from build123d import *

# Parameters (mm, degrees)
F0_R     = 29
F0_R_2   = 20.25
F1_DEPTH = 40
F2_SIZE  = 5
F3_SIZE  = 2
F4_SIZE  = 2
F5_SIZE  = 5


with BuildPart() as f1:
    # F0 (on Top) → F1 (new body, symmetric)
    with BuildSketch(Plane.XY):
        Circle(F0_R)
        Circle(F0_R_2, mode=Mode.SUBTRACT)
    extrude(amount=F1_DEPTH, both=True)

    # F2
    f2_edges = [f1.edges().sort_by_distance(p)[0] for p in [
        (-20.25, 0, 40),
    ]]
    chamfer(f2_edges, length=F2_SIZE)

    # F3
    f3_edges = [f1.edges().sort_by_distance(p)[0] for p in [
        (-29, 0, -40),
    ]]
    chamfer(f3_edges, length=F3_SIZE)

    # F4
    f4_edges = [f1.edges().sort_by_distance(p)[0] for p in [
        (-29, 0, 40),
    ]]
    chamfer(f4_edges, length=F4_SIZE)

    # F5
    f5_edges = [f1.edges().sort_by_distance(p)[0] for p in [
        (-20.25, 0, -40),
    ]]
    chamfer(f5_edges, length=F5_SIZE)


solid = f1.part
Source: CAD feature listing. Evaluate the final solid. Frame: model axes, mm. Coordinates: 2 decimals unless noted, no trailing zeros. Loops run counter-clockwise (first coordinate to the right, second up) from the corner with the lowest first, then second, coordinate; pieces in that order, holes last. Notation, with made-up numbers: (27, 78.5) - (54, 78.5) arc R23 ccw to (54, 106.5) - close; hole circle Ø3 at (64.5, 74). An arc over 180 degrees is marked (long way). Return JSON: item names as keys, results as strings.
Q1. Contact query for flat-ended pins moving along their axis: P1, Ø5, axis at x = 10.5, z = 26.5, coming from the +Y side; P2, Ø5, axis at x = -12, z = 14.5, coming from the +Y side; P3, Ø3, axis at y = -6.5, z = -21.5, coming from the -X side. Output: stop coordinate, or through.
Results:
{"P1": "y = 27.87", "P2": "y = 27.4", "P3": "x = -28.57"}
Q2. Section C-C, the plane z = 29. Return loops of the section in (x, y).
Results:
{"outline": "circle Ø58 at (0, 0); hole circle Ø40.5 at (0, 0)"}
Q3. Mould query, pull axis Y, two halves, no side actions, for faces 1 (the flat face through (18, -18, -40)), 2 (the cylindrical face through (13.38, -25.73, 0.53)), 3 (the cylindrical face through (11, 17, 0)). Classes: released by +Y, released by -Y, zero draft, split by the parting line, or undercut.
Results:
{"face 1": "zero draft", "face 2": "split by the parting line", "face 3": "undercut"}
Q4. Section A-A, the plane x = 0. Return loops of the section in (y, z).
Results:
{"outline": "(-29, -38) - (-27, -40) - (-25.25, -40) - (-20.25, -35) - (-20.25, 35) - (-25.25, 40) - (-27, 40) - (-29, 38) - close; (20.25, -35) - (25.25, -40) - (27, -40) - (29, -38) - (29, 38) - (27, 40) - (25.25, 40) - (20.25, 35) - close"}
Q5. Material intervals for line 1 along Y through (x, z) = (0, 0); line 2 along Y through (x, z) = (-15.5, -19); line 3 along X through (y, z) = (-3, -21), sorted ascending.
Results:
{"line 1": "-29 to -20.25, 20.25 to 29", "line 2": "-24.51 to -13.03, 13.03 to 24.51", "line 3": "-28.84 to -20.03, 20.03 to 28.84"}
